from build123d import *

# Parameters (mm, degrees)
F0_W     = 85
F0_H     = 55
F1_DEPTH = 0.4
F3_DEPTH = 0.4


with BuildPart() as f1:
    # F0 (on Top) → F1 (new body)
    with BuildSketch(Plane.XY):
        Rectangle(F0_W, F0_H)
    extrude(amount=F1_DEPTH)

    # F2 (on face) → F3 (join)
    with BuildSketch(Plane.XY.offset(0.4)):
        with BuildLine():
            Line((-10.172568, 10.256139), (-10.172568, 2.418078))
            Line((-10.172568, 2.418078), (-2.829556, 2.418078))
            Line((-2.829556, 2.418078), (-2.829556, -1.954707))
            Line((-2.829556, -1.954707), (-10.172568, -1.954707))
            Line((-10.172568, -1.954707), (-10.172568, -14.949387))
            Line((-10.172568, -14.949387), (-12.078729, -14.949387))
            ThreePointArc((-12.078729, -14.949387), (7.389782, -17.741787), (19.119597, -1.954707))
            Line((19.119597, -1.954707), (5.381422, -1.954707))
            Line((5.381422, -1.954707), (5.384529, -14.949387))
            Line((5.384529, -14.949387), (0.97045, -14.949387))
            Line((0.97045, -14.949387), (0.97045, 10.256139))
            Line((0.97045, 10.256139), (-10.172568, 10.256139))
        make_face()
        with BuildLine():
            ThreePointArc((-14.586647, 12.514376), (-19.219258, 0), (-14.586647, -12.514376))
            Line((-14.586647, -12.514376), (-14.586647, 12.514376))
        make_face()
        Polygon((14.71059, 2.418078), (14.713768, 10.256139), (5.384529, 10.256139), (5.381422, 2.418078), align=None)
        with BuildLine():
            ThreePointArc((12.416224, 14.670285), (0, 19.219258), (-12.416224, 14.670285))
            Line((-12.416224, 14.670285), (0.97045, 14.670285))
            Line((0.97045, 14.670285), (1.213219, 14.670285))
            Line((1.213219, 14.670285), (12.416224, 14.670285))
        make_face()
    extrude(amount=F3_DEPTH)


solid = f1.part
Input: part model. Units: mm. Frame: model coordinates. A direction names the side the tool comes from. Round coordinates to 2 decimals unless told otherwise and drop trailing zeros. Write each loop counter-clockwise with the first axis right and the second up, starting at its lowest first coordinate (ties: lowest second). Pieces come first, ordered by that corner, then holes.
1) Cut plane D-D (y = 8.5). Return the cut outline in (x, z).
2) Ray query, L1, parallel to X at y = -3.5, z = 0.75; L2, parallel to X at y = 2.5, z = 0.7; L3, parallel to Z at x = 22, y = -15. Return the intervals inside material, ascending.
3) Cut plane B-B (y = 0). Return the cut outline in (x, z), then the cut area to 3 significant figures.
4) Cut plane C-C (x = 26.5). Return the cut outline in (y, z).
5) Reachability of faces 1 (the cylindrical face through (0.19, 19.22, 0.6)), 2 (the cylindrical face through (7.12, -17.85, 0.6)), 3 (the flat face through (0, 16, 0.8)), 4 (the cylindrical face through (-19.22, 0.19, 0.6)) from +Z, -Z, +X, -X, +Y, -Y: full face, straight path, thin tool, end or side. Return the list, or none.
6) Contact query for a flat-ended pin moving along its axis: P1, Ø3, axis at x = 20.5, y = -4.5, coming from the +Z side. Output: stop coordinate, or through.
7) Cut plane A-A (z = 0.65). Return the cut outline in (x, y).
Geometry says:
1. outline: (-42.5, 0) - (42.5, 0) - (42.5, 0.4) - (14.71, 0.4) - (14.71, 0.8) - (5.38, 0.8) - (5.38, 0.4) - (0.97, 0.4) - (0.97, 0.8) - (-10.17, 0.8) - (-10.17, 0.4) - (-14.59, 0.4) - (-14.59, 0.8) - (-17.24, 0.8) - (-17.24, 0.4) - (-42.5, 0.4) - close
2. L1: x = -18.9 to -14.59, -10.17 to 0.97, 5.38 to 18.9
2. L2: x = -19.06 to -14.59, -10.17 to 0.97, 5.38 to 14.71
2. L3: z = 0 to 0.4
3. outline: (-42.5, 0) - (42.5, 0) - (42.5, 0.4) - (0.97, 0.4) - (0.97, 0.8) - (-2.83, 0.8) - (-2.83, 0.4) - (-14.59, 0.4) - (-14.59, 0.8) - (-19.22, 0.8) - (-19.22, 0.4) - (-42.5, 0.4) - close
3. area: 37.4 mm2
4. outline: (-27.5, 0) - (27.5, 0) - (27.5, 0.4) - (-27.5, 0.4) - close
5. face 1: +Z, +Y
5. face 2: +Z, -Y
5. face 3: +Z, +X, -X, +Y, -Y
5. face 4: +Z, -X
6. P1: stops at z = 0.4
7. outline: (-14.59, -12.51) - (-14.59, 12.51) arc R19.22 ccw to start; (-12.42, 14.67) - (12.42, 14.67) arc R19.22 ccw to start; (-12.08, -14.95) arc R19.22 ccw to (19.12, -1.95) - (5.38, -1.95) - (5.38, -14.95) - (0.97, -14.95) - (0.97, 10.26) - (-10.17, 10.26) - (-10.17, 2.42) - (-2.83, 2.42) - (-2.83, -1.95) - (-10.17, -1.95) - (-10.17, -14.95) - close; (5.38, 2.42) - (14.71, 2.42) - (14.71, 10.26) - (5.38, 10.26) - close
